Read the model definition and answer for the solid it produces. Units are mm, in the model's axes. A direction names the side the tool comes from. Give positions to 0.01 mm unless a question says otherwise; leave off trailing zeros. Order: outer loops, then holes, each group sorted by start corner. A loop starts at its lowest first (then second) coordinate and runs counter-clockwise, first axis right, second up. Notation, with made-up numbers: (-8.75, 79) -> (12.25, 79) arc R28 ccw to (12.25, 110) -> close; hole circle Ø1 at (58, 70). An arc over 180 degrees is marked (long way). One line per item, written item: value. Start each with the question number.
from build123d import *

# Parameters (mm, degrees)
PLATE_SKETCH_W                  = 100
PLATE_SKETCH_H                  = 222
PLATE_EXTRUDE_DEPTH             = 10
PRIMARY_SUPPORT_EXTRUDE_DEPTH   = 10
SECONDARY_SUPPORT_EXTRUDE_DEPTH = 10
GRIPPER_EXTRUDE_DEPTH           = 5


with BuildPart() as part:
    # Plate Sketch → Plate Extrude (new body)
    with BuildSketch(Plane.XY):
        Rectangle(PLATE_SKETCH_W, PLATE_SKETCH_H)
    extrude(amount=-PLATE_EXTRUDE_DEPTH)

    # Primary Support Sketch → Primary Support Extrude (add)
    with BuildSketch(Plane(origin=(50, 0, 0), x_dir=(0, 0, -1), z_dir=(1, 0, 0))):
        Polygon((10, 111), (10, 81), (40, 111), align=None)
    primary_support_extrude = extrude(amount=-PRIMARY_SUPPORT_EXTRUDE_DEPTH)

    # Primary Support Mirror: Primary Support Extrude across plane
    add(primary_support_extrude.mirror(Plane.ZX))

    # Secondary Support Sketch → Secondary Support Extrude (add)
    with BuildSketch(Plane.ZY.offset(50)):
        Polygon((-10, 81), (-40, 111), (-10, 111), align=None)
    extrude(amount=-SECONDARY_SUPPORT_EXTRUDE_DEPTH)

    # Gripper Sketch → Gripper Extrude (add)
    with BuildSketch(Plane(origin=(0, 111, 0), x_dir=(1, 0, 0), z_dir=(0, 1, 0))):
        with BuildLine():
            Line((-50, 0), (50, 0))
            Line((50, 0), (50, 100))
            ThreePointArc((50, 100), (0, 150), (-50, 100))
            Line((-50, 100), (-50, 0))
        make_face()
    gripper_extrude = extrude(amount=GRIPPER_EXTRUDE_DEPTH)

    # Gripper Mirror: Gripper Extrude across plane
    add(gripper_extrude.mirror(Plane.ZX))


solid = part.part
Item 1: Flat-ended cylindrical pins translate along their axes: pin 1 (9 mm diameter, centred on y = -93, z = -27, fed in from -X); pin 2 (10 mm diameter, centred on x = -23.5, y = 49.5, fed in from +Z); pin 3 (12 mm diameter, centred on x = 11, y = -70, fed in from -Z). Find the tip coordinate at first contact, or state that the pin passes through.
Item 2: Find section A-A on z = -14.5. Write down the section's boundary in (x, y), then the cut area to 4 significant figures.
Item 3: A tool of negligible diameter and unlimited length cuts with its end or side. For faces 1 (the flat face through (45, 96, -25)), 2 (the flat face through (-1, 111, -81)), 3 (the flat face through (-1, -111, -81)), from which of +Z, -Z, +X, -X, +Y, -Y can it reach the whole face along a straight path? Write none if from no direction.
Item 4: Find section C-C on z = -37.5. Write down the section's boundary in (x, y).
Item 5: Find section D-D on y = -87. Write down the section's boundary in (x, z), then the cut area to 3 significant figures.
Item 6: Find the intervals of material crossed by line 1 (Y direction, x = 13, z = -79.5); line 2 (X direction, y = 106, z = -34); line 3 (Z direction, x = -15, y = -98), in increasing order. Write a range as from..to.
Item 7: For a pull along Y with two mould halves and no side action, classify faces 4 (the flat face through (-1, -116, -76)), 5 (the cylindrical face through (1.099, 113.465, -149.988)), 6 (the flat face through (45, -96, -25)) as +Y half, -Y half, draft (parallel to the pull), parting line (faces both ways), or undercut.
Item 8: Find section B-B on x = 0. Write down the section's boundary in (y, z).
Checks:
1. pin 1: x = 40
1. pin 2: z = 0
1. pin 3: z = -10
2. outline: (-50, -116) -> (50, -116) -> (50, -85.5) -> (40, -85.5) -> (40, -111) -> (-50, -111) -> close; (-50, 85.5) -> (-40, 85.5) -> (-40, 111) -> (40, 111) -> (40, 85.5) -> (50, 85.5) -> (50, 116) -> (-50, 116) -> close
2. area: 1,765 mm2
3. face 1: -Z, +X, -X
3. face 2: -Z
3. face 3: -Z, -X
4. outline: (-50, -116) -> (50, -116) -> (50, -108.5) -> (40, -108.5) -> (40, -111) -> (-50, -111) -> close; (-50, 108.5) -> (-40, 108.5) -> (-40, 111) -> (40, 111) -> (40, 108.5) -> (50, 108.5) -> (50, 116) -> (-50, 116) -> close
5. outline: (-50, -10) -> (40, -10) -> (40, -16) -> (50, -16) -> (50, 0) -> (-50, 0) -> close
5. area: 1,060 mm2
6. line 1: -116..-111, 111..116
6. line 2: -50..-40, 40..50
6. line 3: -10..0
7. face 4: -Y half
7. face 5: draft
7. face 6: undercut
8. outline: (-116, -150) -> (-111, -150) -> (-111, -10) -> (111, -10) -> (111, -150) -> (116, -150) -> (116, 0) -> (-116, 0) -> close
